Design review of the part built by this model. Coordinates are the model's own, in mm. Face numbers are marked on the shaded views. A direction names the side the tool comes from. Coordinates: 2 decimals unless noted, no trailing zeros. Loops run counter-clockwise (first coordinate to the right, second up) from the corner with the lowest first, then second, coordinate; pieces in that order, holes last.
Q1. Add section C-C on z = 19.05. Give the boundary of the cut face in (x, y) (3 decimals).
Q2. Wall thickness on probe 1 along X at (y, z) = (-1.05, 19.05) (3 decimals); probe 2 along Z at (x, y) = (69.85, -2.15) (3 decimals); probe 3 along X at (y, z) = (30, 13.5): over which ranges is each line inside the solid? List them lowest first.
Q3. Machinability: for the marked faces 1, 2 and 3, which of the approach directions +Z, -Z, +X, -X, +Y, -Y give a long, thin tool a straight path to every point of the face, cutting with its end or side? Answer none if there is none.
Q4. Add section B-B on y = 6. Give the boundary of the cut face in (x, z).
Q5. Draft analysis for pull direction Y (two halves, no side actions). For the marked faces 4, 5, 6 and 7, state which applies: released by +Y, released by -Y, zero draft, split by the parting line, or undercut.
Q6. Add section A-A on x = 78.5. Give the boundary of the cut face in (y, z), and give its area (3 significant figures).
Q7. For P1, Ø6.5, axis at x = 46, y = 4, coming from the -Z side; P2, Ø5.5, axis at x = 69.85, z = 19.05, coming from the -Y side, all flat-tipped, find the tip position at first contact; note any pin that passes through.
Q8. Add section D-D on z = 65.5. Give the boundary of the cut face in (x, y).
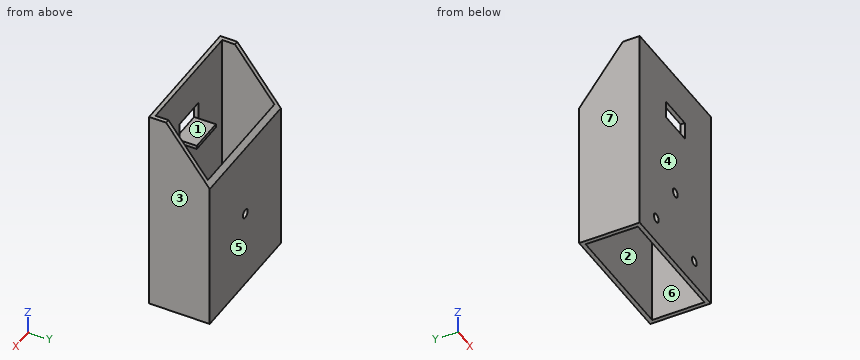
Autodesk Inventor part; units mm, degrees
ref_plane "Work Plane1" through (-3.048, 41.148, 152.4) normal (0, 0.7986, 0.6018) x (-1, 0, 0)
ref_plane "YZ Plane" through (0, 0, 0) normal (1, 0, 0) x (0, 1, 0)
ref_plane "XZ Plane" through (0, 0, 0) normal (0, 1, 0) x (-1, 0, 0)
sketch "Sketch1" plane through (0, 0, 0) normal (0, 0, 1) x (1, 0, 0)
  line L0 (0, 0) -> (88.9, 0)
  line L1 (88.9, 0) -> (88.9, 38.1)
  line L2 (88.9, 38.1) -> (0, 38.1)
  line L3 (0, 38.1) -> (0, 0)
  line L4 (-3.048, 41.148) -> (91.948, 41.148)
  line L5 (91.948, 41.148) -> (91.948, -3.048)
  line L6 (91.948, -3.048) -> (-3.048, -3.048)
  line L7 (-3.048, -3.048) -> (-3.048, 41.148)
  dimension "d0" = 88.9
  dimension "d1" = 38.1
  dimension "d2" = 3.048
extrude "Extrusion1" add sketch "Sketch1" along normal blind 152.4
ref_plane "Work Plane1" through (-3.048, 41.148, 152.4) normal (0, 0.7986, 0.6018) x (-1, 0, 0)
sketch "Sketch2" plane through (-3.048, 41.148, 152.4) normal (0, 0.7986, 0.6018) x (-1, 0, 0)
  line L0 (-144.4625, 77.7875) -> (65.0875, 77.7875)
  line L1 (65.0875, 77.7875) -> (65.0875, -49.2125)
  line L2 (65.0875, -49.2125) -> (-144.4625, -49.2125)
  line L3 (-144.4625, -49.2125) -> (-144.4625, 77.7875)
  point P0 (-3.048, -96.9486)
  dimension "d8" = 127
extrude "Extrusion2" cut sketch "Sketch2" against normal blind 25.4
sketch "Sketch5" plane through (0, 0, 0) normal (0, 1, 0) x (1, 0, 0)
  line L0 (0, 0) -> (0, -152.4)
  line L1 (88.9, -152.4) -> (0, -152.4)
  line L2 (31.75, -110.49) -> (57.15, -110.49)
  line L3 (57.15, -110.49) -> (57.15, -107.95)
  line L4 (57.15, -107.95) -> (31.75, -107.95)
  line L5 (31.75, -107.95) -> (31.75, -110.49)
  line L6 (44.45, -152.4) -> (44.45, -68.5497) construction
  dimension "d21" = 25.4
  dimension "d22" = 2.54
  dimension "d23" = 44.45
  dimension "d24" = 31.75
extrude "Extrusion4" add sketch "Sketch5" along normal blind 12.7
sketch "Sketch7" plane through (0, 0, 0) normal (0, 1, 0) x (1, 0, 0)
  line L0 (57.15, -110.49) -> (31.75, -110.49)
  line L1 (31.75, -110.49) -> (57.15, -110.49)
  line L2 (57.15, -110.49) -> (57.15, -123.19)
  line L3 (57.15, -123.19) -> (31.75, -123.19)
  line L4 (31.75, -123.19) -> (31.75, -110.49)
  dimension "d36" = 12.7
  dimension "d37" = 25.4
  dimension "d38" = 0
extrude "Extrusion5" cut sketch "Sketch7" against normal blind 25.4
sketch "Sketch9" plane through (-3.048, -3.048, 0) normal (0, -1, 0) x (1, 0, 0)
  line L0 (0, 0) -> (0, 152.4)
  line L1 (94.996, 0) -> (0, 0)
  circle A0 centre (22.098, 19.05) radius 3.175
  circle A1 centre (72.898, 19.05) radius 3.175
  point P0 (3.048, 0)
  dimension "d59" = 6.35
  dimension "d60" = 19.05
  dimension "d61" = 22.098
  dimension "d62" = 6.35
  dimension "d63" = 50.8
hole "holePair" at (19.05, -3.048, 19.05) at (69.85, -3.048, 19.05) direction (0, 1, 0) diameter 6.35 depth 25.4 tip angle 118
sketch "Sketch10" plane through (-3.048, -3.048, 0) normal (0, -1, 0) x (1, 0, 0)
  circle A0 centre (22.098, 19.05) radius 3.175
  circle A1 centre (72.898, 19.05) radius 3.175
  line L0 (0, 0) -> (0, 152.4)
  line L1 (22.098, 19.05) -> (72.898, 19.05) construction
  circle A2 centre (47.498, 57.15) radius 3.5015
  point P0 (3.048, 0)
  dimension "d74" = 38.1
hole "Hole5" at (44.45, -3.048, 57.15) direction (0, 1, 0) diameter 6.35 end through all
properties part number "2p1hh" material "Steel, Galvanized"
Entries:
1. outline: (-3.048, -3.048) - (15.875, -3.048) - (15.875, 0) - (0, 0) - (0, 38.1) - (88.9, 38.1) - (88.9, 0) - (73.025, 0) - (73.025, -3.048) - (91.948, -3.048) - (91.948, 41.148) - (-3.048, 41.148) - close; (22.225, -3.048) - (66.675, -3.048) - (66.675, 0) - (22.225, 0) - close
2. probe 1: x = -3.048 to 15.875, 22.225 to 66.675, 73.025 to 91.948
2. probe 2: z = 0 to 15.875, 22.225 to 152.4
2. probe 3: x = -3.05 to 0, 88.9 to 91.95
3. face 1: -Y
3. face 2: +Z, -Z
3. face 3: +Z, -Z, +X, +Y, -Y
4. outline: (-3.05, 0) - (0, 0) - (0, 152.4) - (-3.05, 152.4) - close; (31.75, 107.95) - (57.15, 107.95) - (57.15, 110.49) - (31.75, 110.49) - close; (88.9, 0) - (91.95, 0) - (91.95, 152.4) - (88.9, 152.4) - close
5. face 4: released by -Y
5. face 5: released by +Y
5. face 6: undercut
5. face 7: zero draft
6. outline: (-3.05, 0) - (0, 0) - (0, 152.4) - (-3.05, 152.4) - close; (38.1, 0) - (41.15, 0) - (41.15, 110.19) - (38.1, 114.24) - close
6. area: 807 mm2
7. P1: stops at z = 107.95
7. P2: stops at y = 38.1
8. outline: (-3.05, -3.05) - (91.95, -3.05) - (91.95, 41.15) - (-3.05, 41.15) - close; hole (0, 0) - (88.9, 0) - (88.9, 38.1) - (0, 38.1) - close
